```python
from build123d import *

# Parameters (mm, degrees)
SKETCH1_R           = 1
BOSS_EXTRUDE1_DEPTH = 0.78
SKETCH2_W           = 6.5
SKETCH2_H           = 6.5
BOSS_EXTRUDE2_DEPTH = 6.5
FILLET1_R           = 0.5
SKETCH3_R           = 2.5
BOSS_EXTRUDE3_DEPTH = 6.5
BOSS_EXTRUDE4_DEPTH = 2


with BuildPart() as part:
    # Sketch1 → Boss-Extrude1 (new body)
    with BuildSketch(Plane(origin=(0, 0, 0), x_dir=(1, 0, 0), z_dir=(0, 1, 0))):
        with BuildLine():
            Line((-14.445, -50.065), (14.445, -50.065))
            ThreePointArc((14.445, -50.065), (15.859213562, -49.479213562), (16.445, -48.065))
            Line((16.445, -48.065), (16.445, 48.065))
            ThreePointArc((16.445, 48.065), (15.859213562, 49.479213562), (14.445, 50.065))
            Line((14.445, 50.065), (-14.445, 50.065))
            ThreePointArc((-14.445, 50.065), (-15.859213562, 49.479213562), (-16.445, 48.065))
            Line((-16.445, 48.065), (-16.445, -48.065))
            ThreePointArc((-16.445, -48.065), (-15.859213562, -49.479213562), (-14.445, -50.065))
        make_face()
        with Locations(Location((-13.957298137, 47.395, 0), (0, 0, 90))):
            Circle(SKETCH1_R, mode=Mode.SUBTRACT)
        with Locations(Location((13.752701863, 47.395, 0), (0, 0, 90))):
            Circle(SKETCH1_R, mode=Mode.SUBTRACT)
        with Locations(Location((13.752701863, -47.705, 0), (0, 0, 90))):
            Circle(SKETCH1_R, mode=Mode.SUBTRACT)
        with Locations(Location((-13.957298137, -47.705, 0), (0, 0, 90))):
            Circle(SKETCH1_R, mode=Mode.SUBTRACT)
    extrude(amount=BOSS_EXTRUDE1_DEPTH)

    # Sketch2 → Boss-Extrude2 (add)
    with BuildSketch(Plane(origin=(0, 0.78, 0), x_dir=(1, 0, 0), z_dir=(0, 1, 0))):
        with Locations((-12.145631844, 10.899949454)):
            Rectangle(SKETCH2_W, SKETCH2_H)
    extrude(amount=BOSS_EXTRUDE2_DEPTH)

    # Fillet1
    fillet1_edges = [part.edges().sort_by_distance(p)[0] for p in [
        (-15.395631844, 4.03, -14.149949454),
        (-15.395631844, 4.03, -7.649949454),
        (-8.895631844, 4.03, -7.649949454),
        (-8.895631844, 4.03, -14.149949454),
        (-15.395631844, 7.28, -10.899949454),
        (-12.145631844, 7.28, -7.649949454),
        (-8.895631844, 7.28, -10.899949454),
        (-12.145631844, 7.28, -14.149949454),
    ]]
    fillet(fillet1_edges, radius=FILLET1_R)

    # Sketch3 → Boss-Extrude3 (add)
    with BuildSketch(Plane.ZY.offset(15.395631844)):
        with Locations(Location((-10.899949454, 3.78, 0), (0, 0, 180))):
            Circle(SKETCH3_R)
    extrude(amount=BOSS_EXTRUDE3_DEPTH)

    # Sketch4 → Boss-Extrude4 (add)
    with BuildSketch(Plane(origin=(0, 0.78, 0), x_dir=(1, 0, 0), z_dir=(0, 1, 0))):
        with BuildLine():
            Line((-13.135206183, -10.259829813), (10.737242055, -10.259829813))
            ThreePointArc((10.737242055, -10.259829813), (12.151455617, -10.845616251), (12.737242055, -12.259829813))
            Line((12.737242055, -12.259829813), (12.737242055, -36.056331326))
            ThreePointArc((12.737242055, -36.056331326), (12.151455617, -37.470544888), (10.737242055, -38.056331326))
            Line((10.737242055, -38.056331326), (-13.135206183, -38.056331326))
            ThreePointArc((-13.135206183, -38.056331326), (-14.549419745, -37.470544888), (-15.135206183, -36.056331326))
            Line((-15.135206183, -36.056331326), (-15.135206183, -12.259829813))
            ThreePointArc((-15.135206183, -12.259829813), (-14.549419745, -10.845616251), (-13.135206183, -10.259829813))
        make_face()
    extrude(amount=BOSS_EXTRUDE4_DEPTH)


solid = part.part
```
Model file for the job. Use its own axes, mm. A direction names the side the tool comes from. Coordinates: 2 decimals unless noted, no trailing zeros. Loops run counter-clockwise (first coordinate to the right, second up) from the corner with the lowest first, then second, coordinate; pieces in that order, holes last. Notation, with made-up numbers: (-15.75, 88.25) - (35.25, 88.25) arc R24 ccw to (35.25, 107.25) - close; hole circle Ø3 at (-18.75, 38). An arc over 180 degrees is marked (long way). Answer as a JSON object with one key per item and string values. Group by question number.
(1) Tool access for faces 1 (the face through (-18.6, 3.7, -8.4)), 2 (the face through (-1, 2, 38.056)), 3 (the face through (12.136, 1.766, 10.83)), 4 (the face through (12.17, 1.77, 37.45)), 5 (the face through (12.737, 2, 24)): list every direction of +Z, -Z, +X, -X, +Y, -Y with a clear straight run to the whole face (end or side of a thin tool).
(2) Flat gauge pins, fed straight in: pin 1 (10 mm diameter, centred on x = -8, z = 39.5, fed in from +Y); pin 2 (1.6 mm diameter, centred on y = 1.5, z = 19, fed in from +X) (3 decimals); pin 3 (4 mm diameter, centred on x = 11, z = -18.5, fed in from +Y); pin 4 (2 mm diameter, centred on x = -6.5, y = 2, fed in from +Z). Where does each tip first touch, or does it go through?
(3) Cut at D-D (z = 8.5). Give the cut face in (x, y) (3 decimals), then the cut area to 3 significant figures.
(4) Cut at A-A (y = 3.78). Give the cut face in (x, z), then the cut area to 3 significant figures.
(5) Cut at B-B (z = 28.5). Give the cut face in (x, y) (3 decimals).
(6) Two-plate mould, pull along Z, no slides. Class faces 6 (the face through (15.844, 0.385, 49.495)), 7 (the face through (0, 0, -1)), 8 (the face through (-14.6, 1.8, 10.9)), 9 (the face through (-14.26, 0.38, -48.35)): released by +Z, released by -Z, zero draft, split by the parting line, or undercut.
(7) Cut at C-C (x = -17.5). Give the cut face in (y, z).
(8) Probe line 1 along Y through (x, z) = (4.5, 14.5); line 2 along Y through (x, z) = (-16, -32); line 3 along Z through (x, y) = (-14, 3.5). List the from-to ranges inside material, lowest first.
Geometry says:
{
 "1": {"face 1": "-X", "face 2": "+Z, +X, -X, +Y", "face 3": "-Z, +X, +Y", "face 4": "+Z, +X, +Y", "face 5": "+Z, -Z, +X, +Y"},
 "2": {"pin 1": "stops at y = 2.78", "pin 2": "stops at x = 16.445", "pin 3": "stops at y = 0.78", "pin 4": "stops at z = 38.06"},
 "3": {"outline": "(-16.445, 0) - (16.445, 0) - (16.445, 0.78) - (-16.445, 0.78) - close", "area": "25.7 mm^2"},
 "4": {"outline": "(-21.9, -13.4) - (-15.4, -13.4) - (-15.4, -13.65) arc R0.5 ccw to (-14.9, -14.15) - (-9.4, -14.15) arc R0.5 ccw to (-8.9, -13.65) - (-8.9, -8.15) arc R0.5 ccw to (-9.4, -7.65) - (-14.9, -7.65) arc R0.5 ccw to (-15.4, -8.15) - (-15.4, -8.4) - (-21.9, -8.4) - close", "area": "74.5 mm^2"},
 "5": {"outline": "(-16.445, 0) - (16.445, 0) - (16.445, 0.78) - (12.737, 0.78) - (12.737, 2.78) - (-15.135, 2.78) - (-15.135, 0.78) - (-16.445, 0.78) - close"},
 "6": {"face 6": "released by +Z", "face 7": "zero draft", "face 8": "undercut", "face 9": "undercut"},
 "7": {"outline": "circle Ø5 at (3.78, -10.9)"},
 "8": {"line 1": "y = 0 to 2.78", "line 2": "y = 0 to 0.78", "line 3": "z = -14.15 to -7.65"}
}
